Check sheet for the modelled part. Datum: model origin and axes. Units: mm. A direction names the side the tool comes from. Round coordinates to 2 decimals unless told otherwise and drop trailing zeros. Order: outer loops, then holes, each group sorted by start corner. A loop starts at its lowest first (then second) coordinate and runs counter-clockwise, first axis right, second up.
Q1. Set-up check for faces 5 (the flat face through (37, -1, 50)), 6 (the cylindrical face through (6.32, 20.08, -25.35)), 7 (the cylindrical face through (-17.767, 56.419, 125.35)): record each of +Z, -Z, +X, -X, +Y, -Y from which the full face is reachable in a straight line by a thin tool's end or side.
Q2. Cross-section at A-A on z = -35. Record the cut outline in (x, y), then the cut area to 3 significant figures.
Q3. Scan lines: probe 1 along X at (y, z) = (0, -39.5); probe 2 along X at (y, z) = (0, 116.5); probe 3 along Y at (x, z) = (2.5, 73.5). Record each from-to range of solid material in increasing order.
Q4. Depth check by flat-ended pin: P1, Ø2, axis at x = 18.5, z = 130, coming from the +Y side; P2, Ø0.6, axis at x = -0.5, y = -56, coming from the +Z side; P3, Ø20, axis at x = 29, z = 27.5, coming from the -Y side; P4, Ø2, axis at x = 0, y = 56.5, coming from the +Z side. Enter the tip coordinate at first touch or a pass-through.
Q5. Mould release check, pull along Y, two halves, no side actions. Record for faces 1 (the flat face through (-11, -16, -50)), 2 (the flat face through (-1, -37, 50)), 3 (the conical face through (35.274, -7.833, 39.589)), 4 (the conical face through (26.829, -27.426, 50.7)): +Y half, -Y half, draft (parallel to the pull), parting line (faces both ways), or undercut.
Autodesk Inventor part; units mm, degrees
ref_plane "YZ Plane" through (0, 0, 0) normal (1, 0, 0) x (0, 1, 0)
ref_plane "XZ Plane" through (0, 0, 0) normal (0, 1, 0) x (-1, 0, 0)
ref_plane "XY Plane" through (0, 0, 0) normal (0, 0, 1) x (1, 0, 0)
sketch "Sketch1" plane through (0, 0, 0) normal (1, 0, 0) x (0, 1, 0)
  line L0 (0, 0) -> (19.05, 0)
  line L1 (19.05, 0) -> (57.15, 100)
  line L2 (57.15, 100) -> (0, 100)
  line L3 (0, 100) -> (0, 0)
  line L4 (0, 0) -> (21.05, 0)
  line L5 (0, 100) -> (59.15, 100)
  line L6 (59.15, 100) -> (21.05, 0)
  line L7 (19.05, 0) -> (19.05, -50)
  line L8 (21.05, 0) -> (21.05, -50)
  line L9 (21.05, -50) -> (19.05, -50)
  line L10 (59.15, 100) -> (59.15, 150)
  line L11 (59.15, 150) -> (57.15, 150)
  line L12 (57.15, 150) -> (57.15, 100)
  dimension "d0" = 19.05
  dimension "d1" = 100
  dimension "d2" = 57.15
  dimension "d3" = 21.05
  dimension "d4" = 59.15
  dimension "d5" = 50
  dimension "d6" = 50
revolve "Revolution1" add sketch "Sketch1" angle 360 about axis through (0, 0, 100) along (0, 0, -1) contours L1 L5 L6 L4 | L4 L8 L9 L7 | L12 L11 L10 L5
sketch "Sketch2" plane through (0, 0, 0) normal (1, 0, 0) x (0, 1, 0)
  line L0 (19.05, 0) -> (57.15, 100)
  line L1 (59.15, 100) -> (21.05, 0)
  line L2 (57.15, 100) -> (19.05, 0) construction
  line L3 (55.2811, 100.7121) -> (17.1811, 0.7121)
  line L4 (20.9189, -0.7121) -> (59.0189, 99.2879)
  arc A0 (59.0189, 99.2879) -> (55.2811, 100.7121) centre (57.15, 100) ccw
  arc A1 (17.1811, 0.7121) -> (20.9189, -0.7121) centre (19.05, 0) ccw
  line L5 (-57.15, 100) -> (57.15, 100)
  line L6 (57.15, 100) -> (55.2811, 100.7121)
  line L7 (-19.05, 0) -> (19.05, 0)
  line L8 (19.05, 0) -> (17.1811, 0.7121)
  point P0 (0, 0)
  point P1 (38.1, 50)
  point P2 (55.0098, 100)
  dimension "d8" = 4
extrude "Extrusion1" add sketch "Sketch2" along normal mid plane 2 contours L8 L3 L5 L0
pattern_circular "Circular Pattern1" count 4 over 360 about axis through (0, 0, 125) along (0, 0, -1) of "Extrusion1"
properties part number "4.5 to 1.5 inch reducer"
Results found:
1. face 5: +Z
1. face 6: -Z
1. face 7: +Z, -Z
2. outline: circle Ø42.1 at (0, 0); hole circle Ø38.1 at (0, 0)
2. area: 252 mm2
3. probe 1: x = -21.05 to -19.05, 19.05 to 21.05
3. probe 2: x = -59.15 to -57.15, 57.15 to 59.15
3. probe 3: y = -48.99 to -46.99, 46.99 to 48.99
4. P1: stops at y = 56.5
4. P2: stops at z = 100
4. P3: stops at y = -26.54
4. P4: stops at z = 150
5. face 1: draft
5. face 2: undercut
5. face 3: parting line
5. face 4: undercut
